Verification items for the finished model (mm, model axes). Give positions to 0.01 mm unless a question says otherwise; leave off trailing zeros. Loops run counter-clockwise (first coordinate to the right, second up) from the corner with the lowest first, then second, coordinate; pieces in that order, holes last. Notation, with made-up numbers: M -3,-13 L 8,-13 A8 cw 8,-5 Z; hole C 25,66 d1. An arc over 180 degrees is marked long. Answer in a Markdown table with one row per item.
```python
from build123d import *

# Parameters (mm, degrees)
SKETCH1_W               = 10
SKETCH1_H               = 10
BOSS_EXTRUDE1_DEPTH     = 40
CUT_EXTRUDE1_DEPTH      = 41.620192023
CUT_EXTRUDE1_DEPTH_BACK = 41.620192023
SKETCH2_R               = 2.5


with BuildPart() as part:
    # Sketch1 → Boss-Extrude1 (new, symmetric)
    with BuildSketch(Plane.XY):
        Rectangle(SKETCH1_W, SKETCH1_H)
    extrude(amount=BOSS_EXTRUDE1_DEPTH, both=True)

    # Sketch2 → Cut-Extrude1 (cut, two sides: drawn at the far end of the back side and taken through both)
    with BuildSketch(Plane(origin=(0, 0, 0), x_dir=(1, 0, 0), z_dir=(0, 1, 0)).offset(-CUT_EXTRUDE1_DEPTH_BACK)):
        with Locations(Location((0, -35, 0), (0, 0, 270))):
            Circle(SKETCH2_R)
        with Locations(Location((0, 35, 0), (0, 0, 90))):
            Circle(SKETCH2_R)
    extrude(amount=CUT_EXTRUDE1_DEPTH + CUT_EXTRUDE1_DEPTH_BACK, mode=Mode.SUBTRACT)


solid = part.part
```
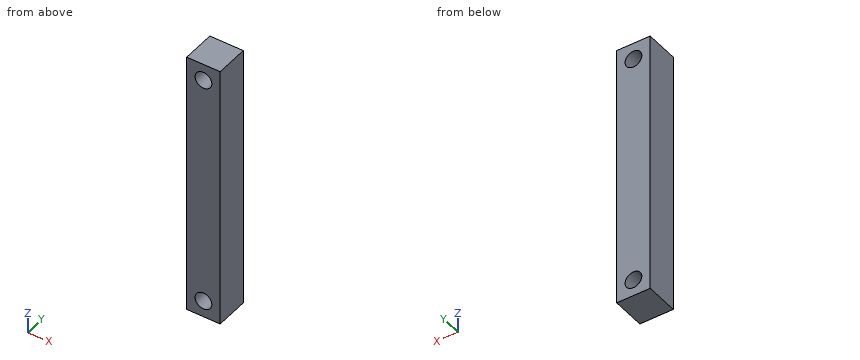
Item 1: Go/stop test with a flat-tipped pin: pin 1 (4.5 mm diameter, centred on x = 0, z = 35, fed in from -Y). Record where the tip stops, or that it passes through.
Reported:
| item | result |
|---|---|
| pin 1 | passes through |
Item 2: Sectioned sample at D-D (z = -34). Record the cut outline in (x, y), and give its area (3 significant figures).
Reported:
| item | result |
|---|---|
| outline | M -5,-5 L -2.29,-5 L -2.29,5 L -5,5 Z; M 2.29,-5 L 5,-5 L 5,5 L 2.29,5 Z |
| area | 54.2 mm^2 |
Item 3: Sectioned sample at A-A (x = 0). Record the cut outline in (y, z), and give its area (3 significant figures).
Reported:
| item | result |
|---|---|
| outline | M -5,-40 L 5,-40 L 5,-37.5 L -5,-37.5 Z; M -5,-32.5 L 5,-32.5 L 5,32.5 L -5,32.5 Z; M -5,37.5 L 5,37.5 L 5,40 L -5,40 Z |
| area | 700 mm^2 |
Item 4: Scan lines: L1, parallel to X at y = -1, z = -35; L2, parallel to Z at x = 0.5, y = -1.5; L3, parallel to Z at x = 1, y = 4.75. Record each from-to range of solid material in increasing order. Write a range as [from, to].
Reported:
| item | result |
|---|---|
| L1 | x = [-5, -2.5], [2.5, 5] |
| L2 | z = [-40, -37.45], [-32.55, 32.55], [37.45, 40] |
| L3 | z = [-40, -37.29], [-32.71, 32.71], [37.29, 40] |
Item 5: Sectioned sample at B-B (z = 35). Record the cut outline in (x, y), and give its area (3 significant figures).
Reported:
| item | result |
|---|---|
| outline | M -5,-5 L -2.5,-5 L -2.5,5 L -5,5 Z; M 2.5,-5 L 5,-5 L 5,5 L 2.5,5 Z |
| area | 50.0 mm^2 |
Item 6: Sectioned sample at C-C (y = 2). Record the cut outline in (x, z), and give its area (3 significant figures).
Reported:
| item | result |
|---|---|
| outline | M -5,-40 L 5,-40 L 5,40 L -5,40 Z; hole C 0,-35 d5; hole C 0,35 d5 |
| area | 761 mm^2 |
